Geometry check sheet. Reference: the model listing, model coordinates, mm. A direction names the side the tool comes from. Round coordinates to 2 decimals unless told otherwise and drop trailing zeros.
```python
from build123d import *

# Parameters (mm, degrees)
SKETCH1_W           = 189.7
SKETCH1_H           = 190
SKETCH1_R           = 1.7
SKETCH1_W_2         = 2.5
SKETCH1_H_2         = 6
BOSS_EXTRUDE1_DEPTH = 10


with BuildPart() as part:
    # Sketch1 → Boss-Extrude1 (new body)
    with BuildSketch(Plane(origin=(0, 0, 0), x_dir=(1, 0, 0), z_dir=(0, 1, 0))):
        with Locations((84.85, 85)):
            Rectangle(SKETCH1_W, SKETCH1_H)
        Circle(SKETCH1_R, mode=Mode.SUBTRACT)
        with Locations((0, 170)):
            Circle(SKETCH1_R, mode=Mode.SUBTRACT)
        with Locations((13.6, 0)):
            Circle(SKETCH1_R, mode=Mode.SUBTRACT)
        with Locations((27.2, 0)):
            Circle(SKETCH1_R, mode=Mode.SUBTRACT)
        with Locations((40.8, 0)):
            Circle(SKETCH1_R, mode=Mode.SUBTRACT)
        with Locations((54.4, 0)):
            Circle(SKETCH1_R, mode=Mode.SUBTRACT)
        with Locations((68, 0)):
            Circle(SKETCH1_R, mode=Mode.SUBTRACT)
        with Locations((81.6, 0)):
            Circle(SKETCH1_R, mode=Mode.SUBTRACT)
        with Locations((95.2, 0)):
            Circle(SKETCH1_R, mode=Mode.SUBTRACT)
        with Locations((108.8, 0)):
            Circle(SKETCH1_R, mode=Mode.SUBTRACT)
        with Locations((122.4, 0)):
            Circle(SKETCH1_R, mode=Mode.SUBTRACT)
        with Locations((136, 0)):
            Circle(SKETCH1_R, mode=Mode.SUBTRACT)
        with Locations((149.6, 0)):
            Circle(SKETCH1_R, mode=Mode.SUBTRACT)
        with Locations((163.2, 0)):
            Circle(SKETCH1_R, mode=Mode.SUBTRACT)
        with Locations((95.2, 170)):
            Circle(SKETCH1_R, mode=Mode.SUBTRACT)
        with Locations((163.2, 170)):
            Circle(SKETCH1_R, mode=Mode.SUBTRACT)
        with Locations((5.25, 105)):
            Rectangle(SKETCH1_W_2, SKETCH1_H_2, mode=Mode.SUBTRACT)
        with Locations((18.85, 105)):
            Rectangle(SKETCH1_W_2, SKETCH1_H_2, mode=Mode.SUBTRACT)
        with Locations((32.45, 105)):
            Rectangle(SKETCH1_W_2, SKETCH1_H_2, mode=Mode.SUBTRACT)
        with Locations((46.05, 105)):
            Rectangle(SKETCH1_W_2, SKETCH1_H_2, mode=Mode.SUBTRACT)
        with Locations((59.65, 105)):
            Rectangle(SKETCH1_W_2, SKETCH1_H_2, mode=Mode.SUBTRACT)
        with Locations((73.25, 105)):
            Rectangle(SKETCH1_W_2, SKETCH1_H_2, mode=Mode.SUBTRACT)
        with Locations((86.85, 105)):
            Rectangle(SKETCH1_W_2, SKETCH1_H_2, mode=Mode.SUBTRACT)
        with Locations((100.45, 105)):
            Rectangle(SKETCH1_W_2, SKETCH1_H_2, mode=Mode.SUBTRACT)
        with Locations((114.05, 105)):
            Rectangle(SKETCH1_W_2, SKETCH1_H_2, mode=Mode.SUBTRACT)
        with Locations((127.65, 105)):
            Rectangle(SKETCH1_W_2, SKETCH1_H_2, mode=Mode.SUBTRACT)
        with Locations((141.25, 105)):
            Rectangle(SKETCH1_W_2, SKETCH1_H_2, mode=Mode.SUBTRACT)
        with Locations((154.85, 105)):
            Rectangle(SKETCH1_W_2, SKETCH1_H_2, mode=Mode.SUBTRACT)
        with Locations((168.45, 105)):
            Rectangle(SKETCH1_W_2, SKETCH1_H_2, mode=Mode.SUBTRACT)
    extrude(amount=-BOSS_EXTRUDE1_DEPTH)


solid = part.part
```
1) Access from +Z, -Z, +X, -X, +Y, -Y to the whole of each face (thin tool, end or side, straight path). Record for faces 1 (the face through (84, 0, -86)), 2 (the face through (44.8, -5, -105)).
Report:
face 1: +Z, -Z, +X, -X, +Y
face 2: +Y, -Y
2) Mould release check, pull along Z, two halves, no side actions. Record for faces 3 (the face through (20.1, -5, -105)), 4 (the face through (179.7, -5, -84)), 5 (the face through (84, -5, -180)): +Z half, -Z half, draft (parallel to the pull), parting line (faces both ways), or undercut.
Report:
face 3: undercut
face 4: draft
face 5: -Z half
3) Scan lines: line 1 along Z through (x, y) = (0, -6.25); line 2 along Z through (x, y) = (96.5, -3); line 3 along Z through (x, y) = (113.5, -1). Record each from-to range of solid material in increasing order.
Report:
line 1: z = -180 to -171.7, -168.3 to -1.7, 1.7 to 10
line 2: z = -180 to -171.1, -168.9 to -1.1, 1.1 to 10
line 3: z = -180 to -108, -102 to 10
4) Gauge pin test, flat end, axial feed: pin 1 (4 mm diameter, centred on x = 136, z = 0, fed in from -Y). Record the tip position at first contact, or that the pin passes through.
Report:
pin 1: stops at y = -10
